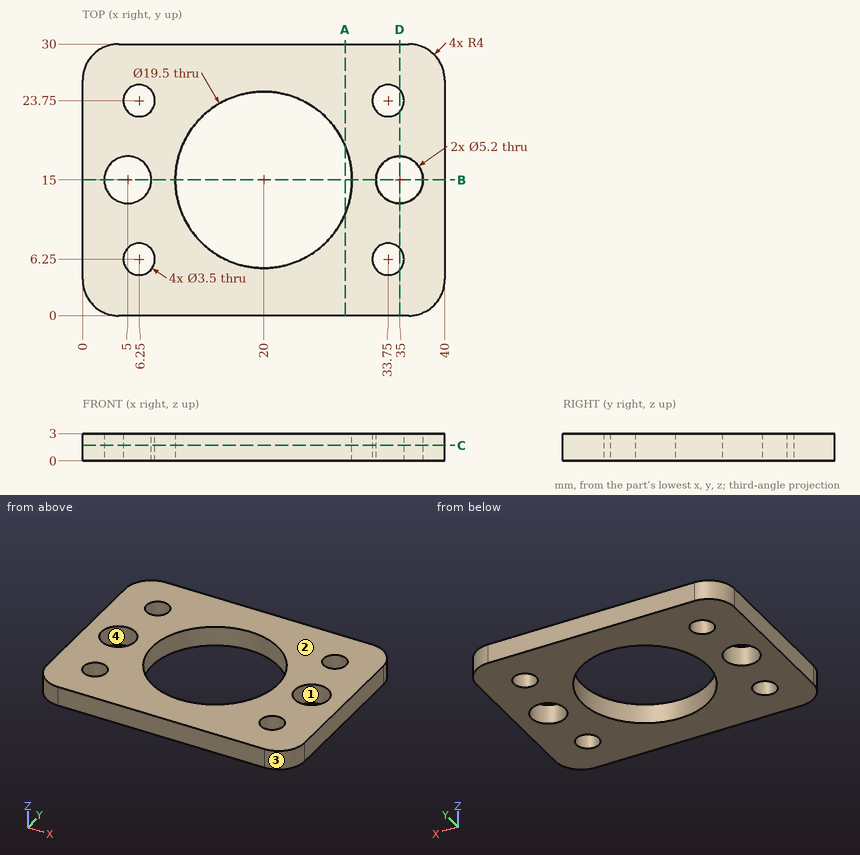
Drawing for the job (mm, zero at the part's lowest x, y, z). Round coordinates to 2 decimals unless told otherwise and drop trailing zeros. Write each loop counter-clockwise with the first axis right and the second up, starting at its lowest first coordinate (ties: lowest second). Pieces come first, ordered by that corner, then holes. Notation, with made-up numbers: M 50.5,28 L 70.5,28 A27 cw 70.5,46 Z; hole C 22.25,65 d1. An arc over 180 degrees is marked long. Answer in a Markdown table with one row per item.
1. Mould opens along Y. For the marked faces 1, 2, 3 and 4 say: +Y half, -Y half, draft (parallel to the pull), parting line (faces both ways), or undercut.
Geometry check:
| item | result |
|---|---|
| face 1 | undercut |
| face 2 | draft |
| face 3 | -Y half |
| face 4 | undercut |
2. Saw through at A-A (x = 29). List the corners of the cut face in (y, z).
Geometry check:
| item | result |
|---|---|
| outline | M 0,0 L 11.25,0 L 11.25,3 L 0,3 Z; M 18.75,0 L 30,0 L 30,3 L 18.75,3 Z |
3. Saw through at D-D (x = 35). List the corners of the cut face in (y, z), and give its area (3 significant figures).
Geometry check:
| item | result |
|---|---|
| outline | M 0,0 L 5.03,0 L 5.03,3 L 0,3 Z; M 7.47,0 L 12.4,0 L 12.4,3 L 7.47,3 Z; M 17.6,0 L 22.53,0 L 22.53,3 L 17.6,3 Z; M 24.97,0 L 30,0 L 30,3 L 24.97,3 Z |
| area | 59.7 mm2 |
4. Saw through at B-B (y = 15). List the corners of the cut face in (x, z), and give its area (3 significant figures).
Geometry check:
| item | result |
|---|---|
| outline | M 0,0 L 2.4,0 L 2.4,3 L 0,3 Z; M 7.6,0 L 10.25,0 L 10.25,3 L 7.6,3 Z; M 29.75,0 L 32.4,0 L 32.4,3 L 29.75,3 Z; M 37.6,0 L 40,0 L 40,3 L 37.6,3 Z |
| area | 30.3 mm2 |
5. Saw through at C-C (z = 1.7). List the corners of the cut face in (x, y), and give its area (3 significant figures).
Geometry check:
| item | result |
|---|---|
| outline | M 0,4 A4 ccw 4,0 L 36,0 A4 ccw 40,4 L 40,26 A4 ccw 36,30 L 4,30 A4 ccw 0,26 Z; hole C 5,15 d5.2; hole C 6.25,6.25 d3.5; hole C 6.25,23.75 d3.5; hole C 20,15 d19.5; hole C 33.75,6.25 d3.5; hole C 33.75,23.75 d3.5; hole C 35,15 d5.2 |
| area | 807 mm2 |
6. Flat gauge pin, fed straight in: P1, Ø11.5, axis at x = 20, y = 15, coming from the -Z side. Where does the tip first touch, or does it go through?
Geometry check:
| item | result |
|---|---|
| P1 | through |
7. Probe L1, parallel to Y at x = 7, z = 1.1; L2, parallel to X at y = 7.25, z = 1.3; L3, parallel to X at y = 23.25, z = 0.8. List the from-to ranges inside material, lowest first. Write a range as [from, to].
Geometry check:
| item | result |
|---|---|
| L1 | [0, 4.67], [7.83, 13.34], [16.66, 22.17], [25.33, 30] |
| L2 | [0, 4.81], [7.69, 14.08], [25.92, 32.31], [35.19, 40] |
| L3 | [0, 4.57], [7.93, 14.8], [25.2, 32.07], [35.43, 40] |
